from build123d import *

# Parameters (mm, degrees)
SKETCH055_W     = 20
SKETCH055_H     = 60
SKETCH055_W_2   = 10
SKETCH055_H_2   = 30
PAD031_DEPTH    = 22
SKETCH056_R     = 1.75
POCKET028_DEPTH = 20.001
POCKET029_DEPTH = 2
SKETCH058_W     = 1
SKETCH058_H     = 22
POCKET030_DEPTH = 11
SKETCH059_W     = 10
SKETCH059_H     = 2
PAD032_DEPTH    = 40


with BuildPart() as part:
    # Sketch055 → Pad031 (new body)
    with BuildSketch(Plane.XZ):
        Rectangle(SKETCH055_W, SKETCH055_H)
        Polygon((1.25, 20.3349364905), (2.5, 22.5), (1.25, 24.6650635095), (-1.25, 24.6650635095), (-2.5, 22.5), (-1.25, 20.3349364905), align=None, mode=Mode.SUBTRACT)
        Polygon((2.5, -22.5), (1.25, -20.3349364905), (-1.25, -20.3349364905), (-2.5, -22.5), (-1.25, -24.6650635095), (1.25, -24.6650635095), align=None, mode=Mode.SUBTRACT)
        Rectangle(SKETCH055_W_2, SKETCH055_H_2, mode=Mode.SUBTRACT)
    extrude(amount=PAD031_DEPTH)

    # Sketch056 (on Face2 of Pad031) → Pocket028 (cut, through all)
    with BuildSketch(Plane(origin=(10, 0, 0), x_dir=(0, 0, 1), z_dir=(1, 0, 0))):
        with Locations((0, 11)):
            Circle(SKETCH056_R)
    extrude(amount=-POCKET028_DEPTH, mode=Mode.SUBTRACT)

    # Sketch057 (on Face2 of Pocket028) → Pocket029 (cut)
    with BuildSketch(Plane(origin=(-10, 0, 0), x_dir=(0, 0, -1), z_dir=(-1, 0, 0))):
        Polygon((2.5980762114, 9.5), (2.5980762114, 12.5), (0, 14), (-2.5980762114, 12.5), (-2.5980762114, 9.5), (0, 8), align=None)
    extrude(amount=-POCKET029_DEPTH, mode=Mode.SUBTRACT)

    # Sketch058 (on Face2 of Pocket029) → Pocket030 (cut)
    with BuildSketch(Plane(origin=(-10, 0, 0), x_dir=(0, 0, -1), z_dir=(-1, 0, 0))):
        with Locations((22.5, 11)):
            Rectangle(SKETCH058_W, SKETCH058_H)
        with Locations((-22.5, 11)):
            Rectangle(SKETCH058_W, SKETCH058_H)
    extrude(amount=-POCKET030_DEPTH, mode=Mode.SUBTRACT)

    # Sketch059 (on Face4 of Pocket030) → Pad032 (join)
    with BuildSketch(Plane(origin=(0, 0, 0), x_dir=(1, 0, 0), z_dir=(0, 1, 0))):
        with Locations((0, 17)):
            Rectangle(SKETCH059_W, SKETCH059_H)
        with Locations((0, -17)):
            Rectangle(SKETCH059_W, SKETCH059_H)
    extrude(amount=PAD032_DEPTH)


solid = part.part
Model file for the job. Use its own axes, mm. A direction names the side the tool comes from. Coordinates: 2 decimals unless noted, no trailing zeros. Order: outer loops, then holes, each group sorted by start corner. A loop starts at its lowest first (then second) coordinate and runs counter-clockwise, first axis right, second up. Notation, with made-up numbers: (44.25, 88) -> (61.25, 88) arc R19 cw to (61.25, 102) -> close; hole circle Ø5 at (15, -9). An arc over 180 degrees is marked (long way). Return JSON: item names as keys, results as strings. Group by question number.
Item 1: Pull direction Y, two halves, no side cores. Call faces 1 (the cylindrical face through (-6.479, -12.735, -0.228)), 2 (the flat face through (-5, -8, 0)): pulls with the +Y half, pulls with the -Y half, needs draft (parallel to the pull), parting line crosses it, or undercut.
Item 2: Saw through at D-D on x = 8. Write the cut outline in (y, z), then the cut area to 3 significant figures.
Item 3: Saw through at A-A on x = 4. Write the cut outline in (y, z).
Item 4: Tool access for faces 3 (the flat face through (-5, 20, 17)), 4 (the flat face through (5, 20, 17)), 5 (the flat face through (-9.01, -13.24, -1.32)), 6 (the flat face through (0, -11, 15)): list every direction of +Z, -Z, +X, -X, +Y, -Y with a clear straight run to the whole face (end or side of a thin tool).
Item 5: Wall check: line 1 along Z through (x, y) = (-5.75, -6.5); line 2 along Z through (x, y) = (-7.05, -11); line 3 along Y through (x, z) = (7.5, 0). Give the ranges that are in metal, low to high. Write a range as [from, to].
Item 6: Flat gauge pins, fed straight in: P1, Ø1.5, axis at x = 6, z = -14, coming from the +Y side; P2, Ø0.6, axis at y = 20.5, z = -17, coming from the +X side; P3, Ø1, axis at y = 13.5, z = 16.5, coming from the -X side. Where does each tip first touch, or does it go through?
Item 7: Saw through at C-C on y = 7.5. Write the cut outline in (x, z).
Item 8: Saw through at B-B on z = -12. Write the cut outline in (x, y), then the cut area to 3 significant figures.
Values found:
{
 "1": {"face 1": "undercut", "face 2": "needs draft"},
 "2": {"outline": "(-22, -30) -> (0, -30) -> (0, 30) -> (-22, 30) -> close; hole circle Ø3.5 at (-11, 0)", "area": "1,310 mm2"},
 "3": {"outline": "(-22, -30) -> (0, -30) -> (0, -18) -> (40, -18) -> (40, -16) -> (0, -16) -> (0, -15) -> (-22, -15) -> close; (-22, 15) -> (0, 15) -> (0, 16) -> (40, 16) -> (40, 18) -> (0, 18) -> (0, 30) -> (-22, 30) -> close"},
 "4": {"face 3": "+Z, -Z, -X, +Y", "face 4": "+Z, -Z, +X, +Y", "face 5": "-X", "face 6": "+Y, -Y"},
 "5": {"line 1": "z = [-30, -23], [-22, 22], [23, 30]", "line 2": "z = [-30, -23], [-22, -1.75], [1.75, 22], [23, 30]", "line 3": "y = [-22, -12.75], [-9.25, 0]"},
 "6": {"P1": "stops at y = 0", "P2": "stops at x = 5", "P3": "stops at x = -5"},
 "7": {"outline": "(-5, -18) -> (5, -18) -> (5, -16) -> (-5, -16) -> close; (-5, 16) -> (5, 16) -> (5, 18) -> (-5, 18) -> close"},
 "8": {"outline": "(-10, -22) -> (-5, -22) -> (-5, 0) -> (-10, 0) -> close; (5, -22) -> (10, -22) -> (10, 0) -> (5, 0) -> close", "area": "220 mm2"}
}
